Geometry: see drawing. Coordinates: mm, zero at the bounding-box minimum. A direction names the side the tool comes from. Give positions to 0.01 mm unless a question says otherwise; leave off trailing zeros. Order: outer loops, then holes, each group sorted by start corner. A loop starts at its lowest first (then second) coordinate and runs counter-clockwise, first axis right, second up. Notation, with made-up numbers: (1.25, -10.5) - (7.25, -10.5) arc R25 cw to (7.25, 25.5) - close; hole circle Ø4 at (51, 5.5). An arc over 180 degrees is marked (long way). One line per item, written item: value. Start each with the question number.
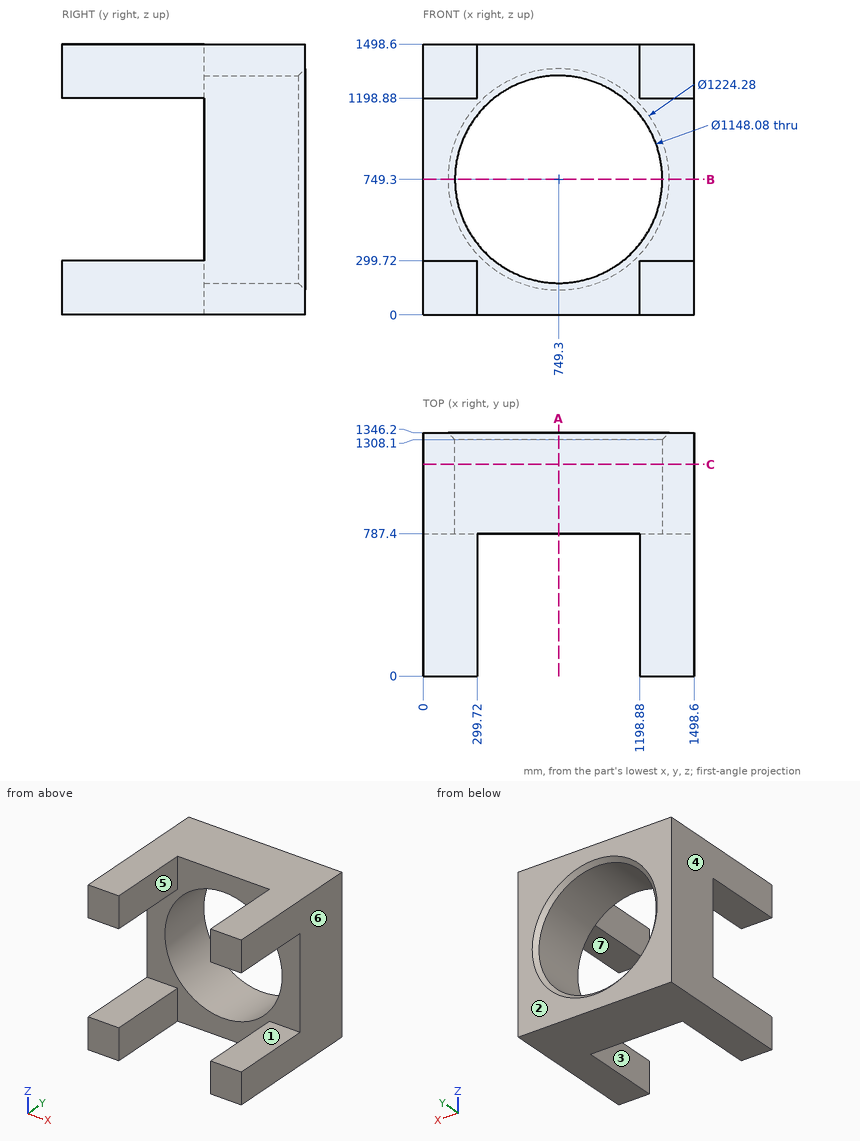
1. Section C-C on y = 1171. Return the cut outline in (x, z), then the cut area to 3 significant figures.
2. Set-up query: the marked faces 1, 2 and 3. Return all of +Z, -Z, +X, -X, +Y, -Y with unobstructed straight access to the full face (end or side cutting, diameter ignored); none if empty.
3. Draft query along X for the marked faces 4, 5, 6 and 7. Return one class per face: pulls with the +X half, pulls with the -X half, needs draft (parallel to the pull), parting line crosses it, or undercut.
4. Section A-A on x = 749.3. Return the cut outline in (y, z).
5. Ray query, L1, parallel to X at y = 1164, z = 749; L2, parallel to Z at x = 70.5, y = 377.5. Return the intervals inside material, ascending.
6. Section B-B on z = 749.3. Return the cut outline in (x, y).
Data:
1. outline: (0, 0) - (1498.6, 0) - (1498.6, 1498.6) - (0, 1498.6) - close; hole circle Ø1148.08 at (749.3, 749.3)
1. area: 1,210,000 mm2
2. face 1: +X, -X, -Y
2. face 2: +Z, -Z, +X, -X, +Y
2. face 3: +Z, -Z, -Y
3. face 4: pulls with the -X half
3. face 5: undercut
3. face 6: pulls with the +X half
3. face 7: needs draft
4. outline: (787.4, 0) - (1346.2, 0) - (1346.2, 137.16) - (1308.1, 175.26) - (787.4, 175.26) - close; (787.4, 1323.34) - (1308.1, 1323.34) - (1346.2, 1361.44) - (1346.2, 1498.6) - (787.4, 1498.6) - close
5. L1: x = 0 to 175.26, 1323.34 to 1498.6
5. L2: z = 0 to 299.72, 1198.88 to 1498.6
6. outline: (0, 787.4) - (175.26, 787.4) - (175.26, 1308.1) - (137.16, 1346.2) - (0, 1346.2) - close; (1323.34, 787.4) - (1498.6, 787.4) - (1498.6, 1346.2) - (1361.44, 1346.2) - (1323.34, 1308.1) - close
